The model under review builds one solid part; all positions refer to its coordinate system, in mm. A direction names the side the tool comes from. Round coordinates to 2 decimals unless told otherwise and drop trailing zeros. Loops run counter-clockwise (first coordinate to the right, second up) from the corner with the lowest first, then second, coordinate; pieces in that order, holes last. Notation, with made-up numbers: M 79.25,83 L 129.25,83 A20 ccw 129.25,104 Z; hole C 86.5,-27 d11. An arc over 180 degrees is marked long. Return JSON: item names as keys, results as strings. Group by question number.
Q1. Consider section C-C (z = -67). State the section outline as (x, y) points (1 decimal), and give its area (3 significant figures).
Q2. Clearance check with flat-ended pins moving along their axes: pin 1 Ø2 at (y, z) = (6.5, -98) entering from -X; pin 2 Ø0.8 at (x, z) = (-0.5, -30.5) entering from -Y; pin 3 Ø1.7 at (y, z) = (10.5, -54) entering from -X. State where each tip first meets the part, or that it passes through.
Q3. Consider section B-B (x = -2.5). State the section outline as (y, z) points (3 decimals), and give its area (3 significant figures).
Q4. For faces 4 (the face through (-1.016, 2, -55)), 5 (the face through (0, 11, -55)), list the 3-axis set-ups (+Z, -Z, +X, -X, +Y, -Y) from which the entire face can be reached by the end or side of a thin tool; tool diameter is ignored.
Q5. To check wall thickness, follow line 1 along X through (y, z) = (2.5, -51.5); line 2 along Y through (x, z) = (-3.5, -25.5); line 3 along X through (y, z) = (9.75, -13.5). State the ranges of each line that lie inside material, in increasing order.
Q6. Draft analysis for pull direction Y (two halves, no side actions). For faces 1 (the face through (-11.112, 2, -55)), 2 (the face through (-5, 0, -55)), 3 (the face through (-6, 1.016, -55)), state which applies: pulls with the +Y half, pulls with the -Y half, needs draft (parallel to the pull), parting line crosses it, or undercut.
Q7. Consider section D-D (y = 7.75). State the section outline as (x, z) points (3 decimals).
Q8. Consider section A-A (y = 2). State the section outline as (x, z) points (1 decimal).
from build123d import *

# Parameters (mm, degrees)
EXTRUDE_THIN1_DEPTH = 111.125
FILLET1_R           = 1.016


with BuildPart() as part:
    # Sketch1 → Extrude-Thin1 (new body)
    with BuildSketch(Plane.XY):
        with BuildLine():
            Line((0, 3.175), (0, 0))
            Line((0, 0), (-11.1125, 0))
            Line((-11.1125, 0), (-11.1125, 3.96875))
            Line((-11.1125, 3.96875), (-8.73125, 3.96875))
            ThreePointArc((-8.73125, 3.96875), (-6.173926083, 10.142676083), (0, 12.7))
            Line((0, 12.7), (0, 9.525))
            Line((0, 9.525), (-1.016, 9.525))
            Line((-1.016, 9.525), (-1.016, 11.616810314))
            ThreePointArc((-1.016, 11.616810314), (-6.1264158, 8.658324821), (-7.648060314, 2.95275))
            Line((-7.648060314, 2.95275), (-10.0965, 2.95275))
            Line((-10.0965, 2.95275), (-10.0965, 1.016))
            Line((-10.0965, 1.016), (-1.016, 1.016))
            Line((-1.016, 1.016), (-1.016, 3.175))
            Line((-1.016, 3.175), (0, 3.175))
        make_face()
    extrude(amount=-EXTRUDE_THIN1_DEPTH)

    # Fillet1
    fillet1_edges = [part.edges().sort_by_distance(p)[0] for p in [
        (-7.648060314, 2.95275, -55.5625),
        (0, 0, -55.5625),
        (-11.1125, 0, -55.5625),
        (-11.1125, 3.96875, -55.5625),
        (0, 12.7, -55.5625),
    ]]
    fillet(fillet1_edges, radius=FILLET1_R)


solid = part.part
Values:
{
 "1": {"outline": "M -11.1,1 A1 ccw -10.1,0 L -1,0 A1 ccw 0,1 L 0,3.2 L -1,3.2 L -1,1 L -10.1,1 L -10.1,3 L -8.7,3 A1 ccw -7.7,4 A7.7 cw -1,11.6 L -1,9.5 L 0,9.5 L 0,11.6 A1 ccw -1.1,12.6 A8.7 ccw -8.7,4 L -10.1,4 A1 ccw -11.1,3 Z", "area": "33.0 mm2"},
 "2": {"pin 1": "stops at x = -8.6", "pin 2": "stops at y = 0.01", "pin 3": "stops at x = -6.63"},
 "3": {"outline": "M 0,-111.125 L 1.016,-111.125 L 1.016,0 L 0,0 Z; M 11.268,-111.125 L 12.334,-111.125 L 12.334,0 L 11.268,0 Z", "area": "231 mm2"},
 "4": {"face 4": "+Z, -Z", "face 5": "+Z, -Z, +X, +Y, -Y"},
 "5": {"line 1": "x = -11.11 to -10.1, -1.02 to 0", "line 2": "y = 0 to 1.02, 10.84 to 11.97", "line 3": "x = -6.54 to -5.11, -1.02 to 0"},
 "6": {"face 1": "needs draft", "face 2": "pulls with the -Y half", "face 3": "undercut"},
 "7": {"outline": "M -7.87,-111.125 L -6.725,-111.125 L -6.725,0 L -7.87,0 Z"},
 "8": {"outline": "M -11.1,-111.1 L -10.1,-111.1 L -10.1,0 L -11.1,0 Z; M -1,-111.1 L 0,-111.1 L 0,0 L -1,0 Z"}
}
